```python
from build123d import *

# Parameters (mm, degrees)
SKETCH2_R           = 2.5
BOSS_EXTRUDE1_DEPTH = 7
SKETCH3_R           = 2.8
BOSS_EXTRUDE2_DEPTH = 0.7
FILLET1_R           = 2.5
SKETCH4_W           = 0.409361502
SKETCH4_H           = 0.4847702
BOSS_EXTRUDE3_DEPTH = 5


with BuildPart() as part:
    # Sketch2 → Boss-Extrude1 (new body)
    with BuildSketch(Plane(origin=(0, 0, 0), x_dir=(1, 0, 0), z_dir=(0, 1, 0))):
        Circle(SKETCH2_R)
    extrude(amount=BOSS_EXTRUDE1_DEPTH)

    # Sketch3 → Boss-Extrude2 (add)
    with BuildSketch(Plane.XZ):
        Circle(SKETCH3_R)
    extrude(amount=BOSS_EXTRUDE2_DEPTH)

    # Fillet1
    fillet1_edges = [part.edges().sort_by_distance(p)[0] for p in [
        (-2.5, 7, 0),
    ]]
    fillet(fillet1_edges, radius=FILLET1_R)

    # Sketch4 → Boss-Extrude3 (add)
    with BuildSketch(Plane.XZ.offset(0.7)):
        with Locations((1.346583888, 0)):
            Rectangle(SKETCH4_W, SKETCH4_H)
        with Locations((-1.346583888, 0)):
            Rectangle(SKETCH4_W, SKETCH4_H)
    extrude(amount=BOSS_EXTRUDE3_DEPTH)


solid = part.part
```
Read the model definition and answer for the solid it produces. Units are mm, in the model's axes. A direction names the side the tool comes from. Give positions to 0.01 mm unless a question says otherwise; leave off trailing zeros. Write each loop counter-clockwise with the first axis right and the second up, starting at its lowest first coordinate (ties: lowest second). Pieces come first, ordered by that corner, then holes. Notation, with made-up numbers: (88, 0.25) -> (96, 0.25) arc R32 cw to (96, 29.25) -> close; hole circle Ø7 at (66, 84). An arc over 180 degrees is marked (long way). Answer as a JSON object with one key per item and string values.
1) Straight lines are drawn through the part: probe 1 along X at (y, z) = (-2, -0.1); probe 2 along Z at (x, y) = (-0.8, 5.75); probe 3 along X at (y, z) = (2, -2.25). For each, find the intervals that lie inside material, in ascending order. Write a range as from..to.
Findings below:
{"probe 1": "x = -1.55..-1.14, 1.14..1.55", "probe 2": "z = -2.01..2.01", "probe 3": "x = -1.09..1.09"}
2) Section B-B on z = 0 is taken. Write down the section's boundary in (x, y), then the cut area to 3 significant figures.
Findings below:
{"outline": "(-2.8, -0.7) -> (-1.55, -0.7) -> (-1.55, -5.7) -> (-1.14, -5.7) -> (-1.14, -0.7) -> (1.14, -0.7) -> (1.14, -5.7) -> (1.55, -5.7) -> (1.55, -0.7) -> (2.8, -0.7) -> (2.8, 0) -> (2.5, 0) -> (2.5, 4.5) arc R2.5 ccw to (-2.5, 4.5) -> (-2.5, 0) -> (-2.8, 0) -> close", "area": "40.3 mm^2"}
3) Section A-A on y = -4.5 is taken. Write down the section's boundary in (x, z).
Findings below:
{"outline": "(-1.55, -0.24) -> (-1.14, -0.24) -> (-1.14, 0.24) -> (-1.55, 0.24) -> close; (1.14, -0.24) -> (1.55, -0.24) -> (1.55, 0.24) -> (1.14, 0.24) -> close"}
4) Flat-ended cylindrical pins translate along their axes: pin 1 Ø1 at (y, z) = (2.5, 0.5) entering from +X; pin 2 Ø3 at (x, y) = (2, -0.5) entering from -Z (3 decimals). Find the tip coordinate at first contact, or state that the pin passes through.
Findings below:
{"pin 1": "stops at x = 2.5", "pin 2": "stops at z = -2.755"}
5) Section C-C on x = 0 is taken. Write down the section's boundary in (y, z).
Findings below:
{"outline": "(-0.7, -2.8) -> (0, -2.8) -> (0, -2.5) -> (4.5, -2.5) arc R2.5 ccw to (4.5, 2.5) -> (0, 2.5) -> (0, 2.8) -> (-0.7, 2.8) -> close"}
6) Section D-D on y = 0.5 is taken. Write down the section's boundary in (x, z).
Findings below:
{"outline": "circle Ø5 at (0, 0)"}
7) A tool of negligible diameter and unlimited length cuts with its end or side. For faces 1 (the cylindrical face through (-0.54, 2.22, 2.44)), 2 (the cylindrical face through (-2.8, -0.3, 0.1)), from which of +Z, -Z, +X, -X, +Y, -Y can it reach the whole face along a straight path? Write none if from no direction.
Findings below:
{"face 1": "+Y", "face 2": "+Y, -Y"}
